from build123d import *

# Parameters (mm, degrees)
SKETCH_1_R      = 1
EXTRUDE_1_DEPTH = 1
SKETCH_1_6_W    = 2
SKETCH_1_6_H    = 1
EXTRUDE_3_DEPTH = 4
EXTRUDE_START   = 3
SKETCH_1_7_W    = 2
SKETCH_1_7_H    = 1
EXTRUDE_4_DEPTH = 1


with BuildPart() as part:
    # Sketch 1 → Extrude 1 (new body)
    with BuildSketch(Plane.XY):
        with BuildLine():
            ThreePointArc((2, 2), (0, 4), (-2, 2))
            Line((-2, 2), (-4, 2))
            Line((-4, 2), (-4, 0))
            Line((-4, 0), (2, 0))
            Line((2, 0), (2, 2))
        make_face()
        with Locations((0, 2)):
            Circle(SKETCH_1_R, mode=Mode.SUBTRACT)
    extrude(amount=EXTRUDE_1_DEPTH)

    # Sketch 1_6 → Extrude 3 (add)
    with BuildSketch(Plane.XY):
        Polygon((2, 0), (2, 1), (0, 1), (-2, 1), (-2, 0), align=None)
        with Locations((-3, 0.5)):
            Rectangle(SKETCH_1_6_W, SKETCH_1_6_H)
    extrude(amount=EXTRUDE_3_DEPTH)

    # Sketch 1_7 → Extrude 4 (add)
    with BuildSketch(Plane.XY.offset(EXTRUDE_START)):
        with BuildLine():
            Line((-4, 2), (-2, 2))
            ThreePointArc((-2, 2), (-2.707106781, 2.292893219), (-3, 3))
            Line((-3, 3), (-4, 3))
            Line((-4, 3), (-4, 2))
        make_face()
        with Locations((-3, 1.5)):
            Rectangle(SKETCH_1_7_W, SKETCH_1_7_H)
    extrude(amount=EXTRUDE_4_DEPTH)


solid = part.part
Work out the finished part from the listing and answer in its coordinate system (mm). A direction names the side the tool comes from. Give positions to 0.01 mm unless a question says otherwise; leave off trailing zeros. Order: outer loops, then holes, each group sorted by start corner. A loop starts at its lowest first (then second) coordinate and runs counter-clockwise, first axis right, second up. Notation, with made-up numbers: M -15,43.25 L 29,43.25 A29 ccw 29,69.25 Z; hole C 83.25,66 d7. An arc over 180 degrees is marked long. Return JSON: item names as keys, results as strings.
Q1. Find section C-C, the plane x = 1.3. Write down the section's boundary in (y, z).
Answer below:
{"outline": "M 0,0 L 3.52,0 L 3.52,1 L 1,1 L 1,4 L 0,4 Z"}
Q2. Find section D-D, the plane z = 2.65. Write down the section's boundary in (x, y).
Answer below:
{"outline": "M -4,0 L 2,0 L 2,1 L -4,1 Z"}
Q3. Find section A-A, the plane z = 0.4. Write down the section's boundary in (x, y), and give its area (3 significant figures).
Answer below:
{"outline": "M -4,0 L 2,0 L 2,2 A2 ccw -2,2 L -4,2 Z; hole C 0,2 d2", "area": "15.1 mm^2"}
Q4. Find section B-B, the plane y = 1.5. Write down the section's boundary in (x, z), and give its area (3 significant figures).
Answer below:
{"outline": "M -4,0 L -0.87,0 L -0.87,1 L -4,1 Z; M -4,3 L -2,3 L -2,4 L -4,4 Z; M 0.87,0 L 2,0 L 2,1 L 0.87,1 Z", "area": "6.27 mm^2"}
Q5. Find the intervals of material crossed by line 1 along Y through (x, z) = (0, 0.45); line 2 along Y through (x, z) = (-2.75, 2.6), in increasing order. Write a range as [from, to].
Answer below:
{"line 1": "y = [0, 1], [3, 4]", "line 2": "y = [0, 1]"}
Q6. The mould has two halves that part along Y. Classify faces 1 (the face through (-0.217, 1.024, 0.493)), 2 (the face through (-3.5, 3, 3.5)), 3 (the face through (-1.71, 0.85, 4)): pulls with the +Y half, pulls with the -Y half, needs draft (parallel to the pull), parting line crosses it, or undercut.
Answer below:
{"face 1": "undercut", "face 2": "pulls with the +Y half", "face 3": "needs draft"}
Q7. Each of these flat-tipped pins is pushed along its axis until it touches: pin 1 (0.9 mm diameter, centred on x = 0, z = 2.5, fed in from +Y); pin 2 (0.5 mm diameter, centred on y = 1.5, z = 3.5, fed in from +X); pin 3 (0.5 mm diameter, centred on x = -3.5, z = 3.5, fed in from +Y). Where does it stop, or does it pass through?
Answer below:
{"pin 1": "stops at y = 1", "pin 2": "stops at x = -2", "pin 3": "stops at y = 3"}
Q8. Which of the six approach directions +Z, -Z, +X, -X, +Y, -Y give full straight-line access (tool end or side, diameter ignored) to faces 4 (the face through (-1, 3, 1)), 5 (the face through (0, 4, 0.5)), 6 (the face through (-2, 1.5, 3.5)), 7 (the face through (-1, 1, 0)), 8 (the face through (-3, 2, 0.5))?
Answer below:
{"face 4": "+X, -X, +Y", "face 5": "+Z, -Z, +Y", "face 6": "+Z, +X, +Y", "face 7": "-Z, +X, -X, +Y, -Y", "face 8": "-Z, -X, +Y"}
